Part model, mm, in its own coordinate system. Face numbers are marked on the shaded views. A direction names the side the tool comes from. Coordinates: 2 decimals unless noted, no trailing zeros. Write each loop counter-clockwise with the first axis right and the second up, starting at its lowest first coordinate (ties: lowest second). Pieces come first, ordered by that corner, then holes. Notation, with made-up numbers: (75.25, 3) - (87.25, 3) arc R24 cw to (87.25, 37) - close; hole circle Ø9 at (75.25, 31). An arc over 180 degrees is marked (long way). Use a Markdown table: item, result.
```python
from build123d import *

# Parameters (mm, degrees)
F2_SIZE2 = 0.75
F2_SIZE  = 0.2
F3_SIZE2 = 0.3
F3_SIZE  = 0.1


with BuildPart() as f1:
    # F0 (on Front) → F1 (revolve)
    with BuildSketch(Plane.XZ):
        Polygon((1.2, 7.7), (0, 7.7), (0, 0), (1.255, 0), (1.255, 1.7), (1.1, 1.7), (1.1, 6), (1.2, 6), align=None)
    revolve(axis=Axis((0, 0, 3.85), (0, 0, -1)))

    # F2
    f2_edges = [f1.edges().sort_by_distance(p)[0] for p in [
        (-1.2, 0, 7.7),
    ]]
    chamfer(f2_edges, length=F2_SIZE, length2=F2_SIZE2)

    # F3
    f3_edges = [f1.edges().sort_by_distance(p)[0] for p in [
        (-1.255, 0, 1.7),
    ]]
    chamfer(f3_edges, length=F3_SIZE, length2=F3_SIZE2)


solid = f1.part
```
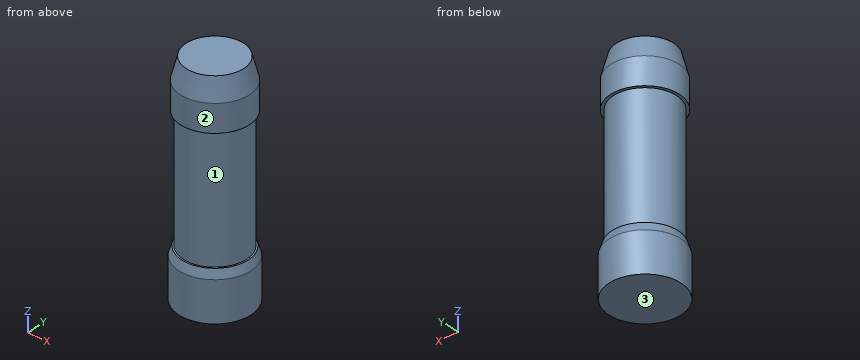
Item 1: Drill centre lines: probe 1 along Y at (x, z) = (0.05, 4.75); probe 2 along X at (y, z) = (-1, 1.25); probe 3 along X at (y, z) = (-0.45, 1.25). Where is each one in solid material? Low to high.
From the geometry:
| item | result |
|---|---|
| probe 1 | -1.1 to 1.1 |
| probe 2 | -0.76 to 0.76 |
| probe 3 | -1.17 to 1.17 |
Item 2: Band-saw the part on A-A, the plane x = 0. Give the cut face in (y, z) (3 decimals), then the cut area to 3 significant figures.
From the geometry:
| item | result |
|---|---|
| outline | (-1.255, 0) - (1.255, 0) - (1.255, 1.4) - (1.155, 1.7) - (1.1, 1.7) - (1.1, 6) - (1.2, 6) - (1.2, 6.95) - (1, 7.7) - (-1, 7.7) - (-1.2, 6.95) - (-1.2, 6) - (-1.1, 6) - (-1.1, 1.7) - (-1.155, 1.7) - (-1.255, 1.4) - close |
| area | 17.6 mm^2 |
Item 3: Which spindle directions (+Z, -Z, +X, -X, +Y, -Y) get a long thin tool onto all of the face, cutting with end or side? Do the marked faces 1, 2 and 3. Say none if no direction does.
From the geometry:
| item | result |
|---|---|
| face 1 | none |
| face 2 | +Z |
| face 3 | -Z, +X, -X, +Y, -Y |
Item 4: Band-saw the part on B-B, the plane z = 4. Give the cut face in (x, y), then the cut area to 3 significant figures.
From the geometry:
| item | result |
|---|---|
| outline | circle Ø2.2 at (0, 0) |
| area | 3.80 mm^2 |
Item 5: Band-saw the part on C-C, the plane z = 6.75. Give the cut face in (x, y).
From the geometry:
| item | result |
|---|---|
| outline | circle Ø2.4 at (0, 0) |
Item 6: Drop a flat-ended pin along its axis: P1, Ø1, axis at x = -1, z = 1, coming from the -Y side. Give the stop position or say it passes through.
From the geometry:
| item | result |
|---|---|
| P1 | y = -1.15 |
